The listing builds one solid part. Answer for the finished solid, in the listing's coordinates (mm). Face numbers are marked on the shaded views. Coordinates: 2 decimals unless noted, no trailing zeros. Loops run counter-clockwise (first coordinate to the right, second up) from the corner with the lowest first, then second, coordinate; pieces in that order, holes last. Notation, with made-up numbers: M 61,-32.5 L 90,-32.5 A16 ccw 90,-2.5 Z; hole C 28.25,59 d2. An arc over 180 degrees is marked long. Answer as a JSON object with one key per item and string values. Group by question number.
1. Determine the mould class of the marked faces 1, 2, 3 and 4 for opening direction Z: released by +Z, released by -Z, zero draft, split by the parting line, or undercut.
2. Straight lines are drawn through the part: L1, parallel to Z at x = 6, y = 9.75; L2, parallel to Y at x = -13, z = -26.67; L3, parallel to Z at x = -1, y = 11.75. For each, find the intervals that lie inside material, in ascending order.
3. A cutting plane is placed at B-B on z = -26.67. Give the vertices of the cut face in (x, y).
4. A cutting plane is placed at C-C on x = -9.5. State how many separate pieces and enclosed holes the cut face has, and give its area (3 significant figures).
5. A cutting plane is placed at A-A on z = 26.67. Give the vertices of the cut face in (x, y).
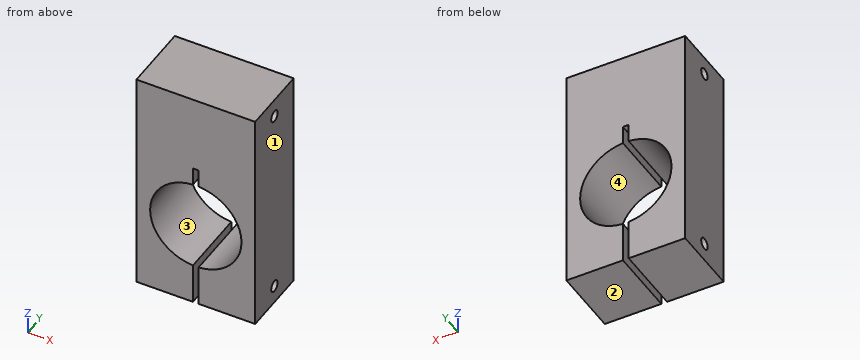
from build123d import *

# Parameters (mm, degrees)
SKETCH1_W           = 33.02
SKETCH1_H           = 63.5
BOSS_EXTRUDE1_DEPTH = 19.05
CUT_EXTRUDE1_DEPTH  = 19.05
SKETCH3_R           = 12.7
CUT_EXTRUDE2_DEPTH  = 19.05
SKETCH4_R           = 1.5875
CUT_EXTRUDE3_DEPTH  = 33.02


with BuildPart() as part:
    # Sketch1 → Boss-Extrude1 (new body)
    with BuildSketch(Plane(origin=(0, 0, 0), x_dir=(1, 0, 0), z_dir=(0, 1, 0))):
        Rectangle(SKETCH1_W, SKETCH1_H)
    extrude(amount=BOSS_EXTRUDE1_DEPTH)

    # Sketch2 → Cut-Extrude1 (cut)
    with BuildSketch(Plane(origin=(0, 19.05, 0), x_dir=(1, 0, 0), z_dir=(0, 1, 0))):
        Polygon((0, 31.75), (0.79375, 31.75), (0.79375, -10.16), (-0.79375, -10.16), (-0.79375, 31.75), align=None)
    extrude(amount=-CUT_EXTRUDE1_DEPTH, mode=Mode.SUBTRACT)

    # Sketch3 → Cut-Extrude2 (cut)
    with BuildSketch(Plane(origin=(0, 19.05, 0), x_dir=(1, 0, 0), z_dir=(0, 1, 0))):
        with Locations((0, 7.62)):
            Circle(SKETCH3_R)
    extrude(amount=-CUT_EXTRUDE2_DEPTH, mode=Mode.SUBTRACT)

    # Sketch4 → Cut-Extrude3 (cut)
    with BuildSketch(Plane(origin=(16.51, 0, 0), x_dir=(0, 0, -1), z_dir=(1, 0, 0))):
        with Locations((-26.67, 9.525)):
            Circle(SKETCH4_R)
        with Locations((26.67, 9.525)):
            Circle(SKETCH4_R)
    extrude(amount=-CUT_EXTRUDE3_DEPTH, mode=Mode.SUBTRACT)


solid = part.part
From the geometry:
{
 "1": {"face 1": "zero draft", "face 2": "released by -Z", "face 3": "undercut", "face 4": "undercut"},
 "2": {"L1": "z = -31.75 to -28.24, -25.1 to -18.81, 3.57 to 25.1, 28.24 to 31.75", "L2": "y = 0 to 7.94, 11.11 to 19.05", "L3": "z = -31.75 to -20.28, 5.04 to 31.75"},
 "3": {"outline": "M -16.51,0 L -0.79,0 L -0.79,7.94 L -16.51,7.94 Z; M -16.51,11.11 L -0.79,11.11 L -0.79,19.05 L -16.51,19.05 Z; M 0.79,0 L 16.51,0 L 16.51,7.94 L 0.79,7.94 Z; M 0.79,11.11 L 16.51,11.11 L 16.51,19.05 L 0.79,19.05 Z"},
 "4": {"separate pieces": "2", "enclosed holes": "2", "area": "873 mm²"},
 "5": {"outline": "M -16.51,0 L 16.51,0 L 16.51,7.94 L -16.51,7.94 Z; M -16.51,11.11 L 16.51,11.11 L 16.51,19.05 L -16.51,19.05 Z"}
}
